The model under review builds one solid part; all positions refer to its coordinate system, in mm. A direction names the side the tool comes from. Round coordinates to 2 decimals unless told otherwise and drop trailing zeros. Loops run counter-clockwise (first coordinate to the right, second up) from the corner with the lowest first, then second, coordinate; pieces in that order, holes last. Notation, with made-up numbers: (49, 37.25) -> (106, 37.25) arc R12 cw to (106, 54.25) -> close; hole circle Ø7 at (-4.5, 48). An arc over 180 degrees is marked (long way). Use a Markdown table: item, result. Add a question column.
1) Consider section A-A on y = -8.5. Give the boundary of the cut face in (x, z), plus the area to 3 significant figures.
2) Consider section B-B on z = 3. Give the boundary of the cut face in (x, y), plus the area to 3 significant figures.
3) Wall thickness on probe 1 along Y at (x, z) = (35, 19); probe 2 along Z at (x, y) = (48, -12.5); probe 3 along X at (y, z) = (-8, 22): over which ranges is each line inside the solid? List them lowest first.
4) Consider section D-D on y = -16.5. Give the boundary of the cut face in (x, z).
5) Consider section C-C on x = 28.5. Give the boundary of the cut face in (y, z).
6) Insertion check: pin 1 (12 mm diameter, centred on x = 31, y = -22.5, fed in from +Z); pin 2 (6.5 mm diameter, centred on x = 44.5, y = -6.5, fed in from +Z). Each pin has a flat end and moves straight along its axis. Give the tip position at first contact, or say it passes through.
7) For faces 1 (the flat face through (45, -12.7, 14)), 2 (the flat face through (19, -25.4, 13)), 3 (the flat face through (41, -6, 19.05)), list the 3-axis set-ups (+Z, -Z, +X, -X, +Y, -Y) from which the entire face can be reached by the end or side of a thin tool; tool diameter is ignored.
from build123d import *

# Parameters (mm, degrees)
F0_W     = 50.8
F0_H     = 31.75
F1_DEPTH = 25.4
F3_DEPTH = 12.7
F5_DEPTH = 25.4


with BuildPart() as f1:
    # F0 (on Front) → F1 (new body)
    with BuildSketch(Plane.XZ):
        with Locations((25.4, 15.875)):
            Rectangle(F0_W, F0_H)
    extrude(amount=F1_DEPTH)

    # F2 (on face) → F3 (cut)
    with BuildSketch(Plane.XZ.offset(25.4)):
        Polygon((50.8, 31.75), (19.05, 31.75), (50.8, 0), align=None)
    extrude(amount=-F3_DEPTH, mode=Mode.SUBTRACT)

    # F4 (on face) → F5 (cut)
    with BuildSketch(Plane.XZ.offset(12.7)):
        Polygon((19.05, 31.75), (31.75, 19.05), (50.8, 19.05), (50.8, 31.75), align=None)
    extrude(amount=-F5_DEPTH, mode=Mode.SUBTRACT)


solid = f1.part
Result set:
| question | item | result |
|---|---|---|
| 1 | outline | (0, 0) -> (50.8, 0) -> (50.8, 19.05) -> (31.75, 19.05) -> (19.05, 31.75) -> (0, 31.75) -> close |
| 1 | area | 1,290 mm2 |
| 2 | outline | (0, -25.4) -> (47.8, -25.4) -> (47.8, -12.7) -> (50.8, -12.7) -> (50.8, 0) -> (0, 0) -> close |
| 2 | area | 1,250 mm2 |
| 3 | probe 1 | -12.7 to 0 |
| 3 | probe 2 | 0 to 19.05 |
| 3 | probe 3 | 0 to 28.8 |
| 4 | outline | (0, 0) -> (50.8, 0) -> (19.05, 31.75) -> (0, 31.75) -> close |
| 5 | outline | (-25.4, 0) -> (0, 0) -> (0, 22.3) -> (-25.4, 22.3) -> close |
| 6 | pin 1 | z = 25.8 |
| 6 | pin 2 | z = 19.05 |
| 7 | face 1 | +Z, +X, -Y |
| 7 | face 2 | +Z, -Z, +X, -X, -Y |
| 7 | face 3 | +Z, +X, +Y, -Y |
